```python
from build123d import *

# Parameters (mm, degrees)
SKETCH1_R           = 2
SKETCH1_R_2         = 3
BOSS_EXTRUDE1_DEPTH = 5
SKETCH1_3_R         = 1.74625
BOSS_EXTRUDE2_DEPTH = 15
FILLET1_R           = 3


with BuildPart() as part:
    # Sketch1 → Boss-Extrude1 (new body)
    with BuildSketch(Plane.XY):
        with BuildLine():
            Line((10, -24.8), (10, -6.25))
            Line((10, -6.25), (-10, -6.25))
            Line((-10, -6.25), (-10, -24.8))
            ThreePointArc((-10, -24.8), (0, -34.8), (10, -24.8))
        make_face()
        with Locations((0, -24.8)):
            Circle(SKETCH1_R, mode=Mode.SUBTRACT)
        with Locations((0, -12.5)):
            Circle(SKETCH1_R_2, mode=Mode.SUBTRACT)
    extrude(amount=BOSS_EXTRUDE1_DEPTH)

    # Sketch1<3> → Boss-Extrude2 (add)
    with BuildSketch(Plane.XY):
        with BuildLine():
            Line((10, -6.25), (10, 0))
            ThreePointArc((10, 0), (0, 10), (-10, 0))
            Line((-10, 0), (-10, -6.25))
            Line((-10, -6.25), (10, -6.25))
        make_face()
        Circle(SKETCH1_3_R, mode=Mode.SUBTRACT)
    extrude(amount=BOSS_EXTRUDE2_DEPTH)

    # Fillet1
    fillet1_edges = [part.edges().sort_by_distance(p)[0] for p in [
        (-10, -6.25, 10),
        (10, -6.25, 10),
    ]]
    fillet(fillet1_edges, radius=FILLET1_R)


solid = part.part
```
Check sheet for the modelled part. Datum: model origin and axes. Units: mm. A direction names the side the tool comes from. Coordinates: 2 decimals unless noted, no trailing zeros. Order: outer loops, then holes, each group sorted by start corner. A loop starts at its lowest first (then second) coordinate and runs counter-clockwise, first axis right, second up. Notation, with made-up numbers: M 64.5,40.5 L 78.5,40.5 A19 ccw 78.5,49.5 Z; hole C 0.25,51 d10. An arc over 180 degrees is marked long. One line per question, with ' | ' between items. Start each with the question number.
Item 1: Sectioned sample at A-A on x = 0. Record the cut outline in (y, z).
Item 2: Gauge pin test, flat ends, axial feed: P1, Ø6, axis at x = -1.5, y = -18.5, coming from the +Z side; P2, Ø5, axis at x = 0, y = -12.5, coming from the +Z side; P3, Ø1, axis at x = -1.5, z = 8, coming from the +Y side. Record the tip position at first contact, or that the pin passes through.
Item 3: Sectioned sample at B-B on z = 11.25. Record the cut outline in (x, y), and give its area (3 significant figures).
Item 4: Mould release check, pull along X, two halves, no side actions. Record for faces 5 (the cylindrical face through (-0.23, 1.73, 7.4)), 6 (the flat face through (10, -10, 4)), 7 (the cylindrical face through (-0.2, -34.8, 2.5)): pulls with the +X half, pulls with the -X half, needs draft (parallel to the pull), parting line crosses it, or undercut.
Item 5: Sectioned sample at C-C on z = 3. Record the cut outline in (x, y), and give its area (3 significant figures).
Item 6: Sectioned sample at D-D on x = -5.5. Record the cut outline in (y, z), and give its area (3 significant figures).
Item 7: Access from +Z, -Z, +X, -X, +Y, -Y to the whole of each face (thin tool, end or side, straight path). Record for faces 1 (the cylindrical face through (9.14, -5.35, 10.07)), 2 (the cylindrical face through (-9.14, -5.35, 10.07)), 3 (the flat face through (0, -6.25, 10)), 4 (the flat face through (-10, -9, 4)).
Item 8: Material ranges on line 1 (Y direction, x = 0, z = 3.75); line 2 (Y direction, x = 0, z = 6.5); line 3 (Z direction, x = 8.5, y = -19), recorded low to high.
Answer below:
1) outline: M -34.8,0 L -26.8,0 L -26.8,5 L -34.8,5 Z; M -22.8,0 L -15.5,0 L -15.5,5 L -22.8,5 Z; M -9.5,0 L -1.75,0 L -1.75,15 L -6.25,15 L -6.25,5 L -9.5,5 Z; M 1.75,0 L 10,0 L 10,15 L 1.75,15 Z
2) P1: stops at z = 5 | P2: passes through | P3: stops at y = 9.95
3) outline: M -10,-3.25 A3 ccw -7,-6.25 L 7,-6.25 A3 ccw 10,-3.25 L 10,0 A10 ccw -10,0 Z; hole C 0,0 d3.49 | area: 269 mm^2
4) face 5: undercut | face 6: pulls with the +X half | face 7: parting line crosses it
5) outline: M -10,-24.8 A10 ccw 10,-24.8 L 10,0 A10 ccw -10,0 Z; hole C 0,-12.5 d6; hole C 0,-24.8 d4; hole C 0,0 d3.49 | area: 760 mm^2
6) outline: M -33.15,0 L 8.35,0 L 8.35,15 L -6.25,15 L -6.25,5 L -33.15,5 Z | area: 354 mm^2
7) face 1: +Z, +X, -Y | face 2: +Z, -X, -Y | face 3: +Z, +X, -X, -Y | face 4: +Z, -Z, -X, +Y, -Y
8) line 1: y = -34.8 to -26.8, -22.8 to -15.5, -9.5 to -1.75, 1.75 to 10 | line 2: y = -6.25 to -1.75, 1.75 to 10 | line 3: z = 0 to 5
